Geometry: final body of the model. Coordinates: model frame, mm. A direction names the side the tool comes from. Round coordinates to 2 decimals unless told otherwise and drop trailing zeros. Write each loop counter-clockwise with the first axis right and the second up, starting at its lowest first coordinate (ties: lowest second). Pieces come first, ordered by that corner, then holes. Notation, with made-up numbers: (-9, 7.25) -> (14, 7.25) arc R25 ccw to (14, 26.25) -> close; hole circle Ø8 at (42, -24). An arc over 180 degrees is marked (long way). Use one line per item in the form item = value. Start each with the question number.
1. Cut plane D-D, the plane z = 0.7. Return the cut outline in (x, y).
2. Cut plane B-B, the plane x = 5. Return the cut outline in (y, z).
3. Line query: L1, parallel to Y at x = 5, z = 0.8; L2, parallel to Y at x = 25, z = 0.6; L3, parallel to X at y = 19.5, z = 0.1. Output: solid intervals per line, ascending.
4. Reachability of faces 1 (the face through (10, 19.9, 0.5)), 2 (the face through (14.8, 0, 0.5)) from +Z, -Z, +X, -X, +Y, -Y: full face, straight path, thin tool, end or side. Return the list, or none.
5. Pin query (flat end, axial travel): pin 1 Ø0.5 at (y, z) = (18.5, 0.5) entering from +X. Return the tip coordinate at first contact, or that it passes through.
6. Cut plane A-A, the plane x = 25. Return the cut outline in (y, z).
7. Draft query along X for faces 3 (the face through (0, 15.2, 0.5)), 4 (the face through (20.1, 10, 0.5)), 5 (the face through (6.386, 14.425, 0.507)). Return one class per face: pulls with the +X half, pulls with the -X half, needs draft (parallel to the pull), parting line crosses it, or undercut.
```python
from build123d import *

# Parameters (mm, degrees)
BOSS_EXTRU_1_DEPTH      = 1
ESQUISSE2_R             = 1.5
ENL_V_MAT_EXTRU_1_DEPTH = 2


with BuildPart() as part:
    # Esquisse1 → Boss.-Extru.1 (new body)
    with BuildSketch(Plane.XY):
        Polygon((0, 0), (30, 0), (30, 10), (10, 10), (10, 30), (0, 30), align=None)
    extrude(amount=BOSS_EXTRU_1_DEPTH)

    # Esquisse2 → Enlèv. mat.-Extru.1 (cut, through all)
    with BuildSketch(Plane.XY.offset(1)):
        with Locations((5, 5)):
            Circle(ESQUISSE2_R)
        with Locations((5, 15)):
            Circle(ESQUISSE2_R)
        with Locations((5, 25)):
            Circle(ESQUISSE2_R)
        with Locations((15, 5)):
            Circle(ESQUISSE2_R)
        with Locations((25, 5)):
            Circle(ESQUISSE2_R)
    extrude(amount=-ENL_V_MAT_EXTRU_1_DEPTH, mode=Mode.SUBTRACT)


solid = part.part
```
Outcome:
q1.outline = (0, 0) -> (30, 0) -> (30, 10) -> (10, 10) -> (10, 30) -> (0, 30) -> close; hole circle Ø3 at (5, 5); hole circle Ø3 at (5, 15); hole circle Ø3 at (5, 25); hole circle Ø3 at (15, 5); hole circle Ø3 at (25, 5)
q2.outline = (0, 0) -> (3.5, 0) -> (3.5, 1) -> (0, 1) -> close; (6.5, 0) -> (13.5, 0) -> (13.5, 1) -> (6.5, 1) -> close; (16.5, 0) -> (23.5, 0) -> (23.5, 1) -> (16.5, 1) -> close; (26.5, 0) -> (30, 0) -> (30, 1) -> (26.5, 1) -> close
q3.L1 = 0 to 3.5, 6.5 to 13.5, 16.5 to 23.5, 26.5 to 30
q3.L2 = 0 to 3.5, 6.5 to 10
q3.L3 = 0 to 10
q4.face_1 = +Z, -Z, +X, +Y
q4.face_2 = +Z, -Z, +X, -X, -Y
q5.pin_1 = 10
q6.outline = (0, 0) -> (3.5, 0) -> (3.5, 1) -> (0, 1) -> close; (6.5, 0) -> (10, 0) -> (10, 1) -> (6.5, 1) -> close
q7.face_3 = pulls with the -X half
q7.face_4 = needs draft
q7.face_5 = undercut
